from build123d import *

# Parameters (mm, degrees)
BOSS_EXTRUDE1_DEPTH = 3.175
SKETCH2_R           = 2.65
CUT_EXTRUDE1_DEPTH  = 94.99510958
FILLET1_R           = 5


with BuildPart() as part:
    # Sketch1 → Boss-Extrude1 (new body)
    with BuildSketch(Plane.XY):
        Polygon((-10, -85), (10, -85), (40, -20), (40, 0), (-40, 0), (-40, -20), align=None)
    extrude(amount=BOSS_EXTRUDE1_DEPTH)

    # Sketch2 → Cut-Extrude1 (cut, through all)
    with BuildSketch(Plane.XY.offset(3.175)):
        with Locations((0, -10)):
            Circle(SKETCH2_R)
        with Locations((30, -10)):
            Circle(SKETCH2_R)
        with Locations((0, -40)):
            Circle(SKETCH2_R)
        with Locations((0, -70)):
            Circle(SKETCH2_R)
        with Locations(Location((-30, -10, 0), (0, 0, 180))):
            Circle(SKETCH2_R)
    extrude(amount=-CUT_EXTRUDE1_DEPTH, mode=Mode.SUBTRACT)

    # Fillet1
    fillet1_edges = [part.edges().sort_by_distance(p)[0] for p in [
        (-40, -20, 1.5875),
        (-40, 0, 1.5875),
        (40, 0, 1.5875),
        (40, -20, 1.5875),
        (10, -85, 1.5875),
        (-10, -85, 1.5875),
    ]]
    fillet(fillet1_edges, radius=FILLET1_R)


solid = part.part
Geometry: final body of the model. Coordinates: model frame, mm. Coordinates: 2 decimals unless noted, no trailing zeros. Order: outer loops, then holes, each group sorted by start corner. A loop starts at its lowest first (then second) coordinate and runs counter-clockwise, first axis right, second up.
(1) Material intervals for probe 1 along Y at (x, z) = (0, 1.4); probe 2 along Y at (x, z) = (-32, 0.25); probe 3 along X at (y, z) = (-68.5, 2.2), sorted ascending.
(2) Section query B-B (z = 1.1). Return the cut outline in (x, y), plus the area to 3 significant figures.
(3) Section query C-C (x = 0). Return the cut outline in (y, z) (3 decimals), plus the area to 3 significant figures.
(4) Section query A-A (y = -10). Return the cut outline in (x, z) (3 decimals).
(5) Section query D-D (y = -40). Return the cut outline in (x, z) (3 decimals), plus the area to 3 significant figures.
Solution:
1. probe 1: y = -85 to -72.65, -67.35 to -42.65, -37.35 to -12.65, -7.35 to 0
1. probe 2: y = -37.33 to -11.74, -8.26 to 0
1. probe 3: x = -17.62 to -2.18, 2.18 to 17.62
2. outline: (-40, -18.9) arc R5 ccw to (-39.54, -21) - (-11.34, -82.1) arc R5 ccw to (-6.8, -85) - (6.8, -85) arc R5 ccw to (11.34, -82.1) - (39.54, -21) arc R5 ccw to (40, -18.9) - (40, -5) arc R5 ccw to (35, 0) - (-35, 0) arc R5 ccw to (-40, -5) - close; hole circle Ø5.3 at (-30, -10); hole circle Ø5.3 at (0, -70); hole circle Ø5.3 at (0, -40); hole circle Ø5.3 at (0, -10); hole circle Ø5.3 at (30, -10)
2. area: 4,730 mm2
3. outline: (-85, 0) - (-72.65, 0) - (-72.65, 3.175) - (-85, 3.175) - close; (-67.35, 0) - (-42.65, 0) - (-42.65, 3.175) - (-67.35, 3.175) - close; (-37.35, 0) - (-12.65, 0) - (-12.65, 3.175) - (-37.35, 3.175) - close; (-7.35, 0) - (0, 0) - (0, 3.175) - (-7.35, 3.175) - close
3. area: 219 mm2
4. outline: (-40, 0) - (-32.65, 0) - (-32.65, 3.175) - (-40, 3.175) - close; (-27.35, 0) - (-2.65, 0) - (-2.65, 3.175) - (-27.35, 3.175) - close; (2.65, 0) - (27.35, 0) - (27.35, 3.175) - (2.65, 3.175) - close; (32.65, 0) - (40, 0) - (40, 3.175) - (32.65, 3.175) - close
5. outline: (-30.769, 0) - (-2.65, 0) - (-2.65, 3.175) - (-30.769, 3.175) - close; (2.65, 0) - (30.769, 0) - (30.769, 3.175) - (2.65, 3.175) - close
5. area: 179 mm2
